Solid Edge part; units mm, degrees
sketch "Sketch1" plane through (0, 0, 0) normal (0, 0, 1) x (1, 0, 0)
  line L0 (-8.89, 16.51) -> (8.89, 16.51)
  line L1 (8.89, 16.51) -> (8.89, -16.51)
  line L2 (8.89, -16.51) -> (-8.89, -16.51)
  line L3 (-8.89, -16.51) -> (-8.89, 16.51)
extrude "Protrusion1" add sketch "Sketch1" along normal blind 1.5875
sketch "Sketch2" plane through (0, 0, 1.5875) normal (0, 0, 1) x (1, 0, 0)
  circle A0 centre (7.62, -15.24) radius 0.4445
  circle A1 centre (4.572, -8.89) radius 0.4445
  circle A2 centre (4.572, -5.9055) radius 0.4445
  circle A3 centre (4.572, 1.27) radius 0.4445
  circle A4 centre (4.572, 3.81) radius 0.4445
  circle A5 centre (7.62, 12.5407) radius 0.4445
  circle A6 centre (6.35, 15.24) radius 0.4445
  circle A7 centre (-6.35, 15.24) radius 0.4445
  circle A8 centre (-7.62, 12.7) radius 0.4445
  circle A9 centre (-7.62, -15.24) radius 0.4445
extrude "Cutout1" cut sketch "Sketch2" against normal through all
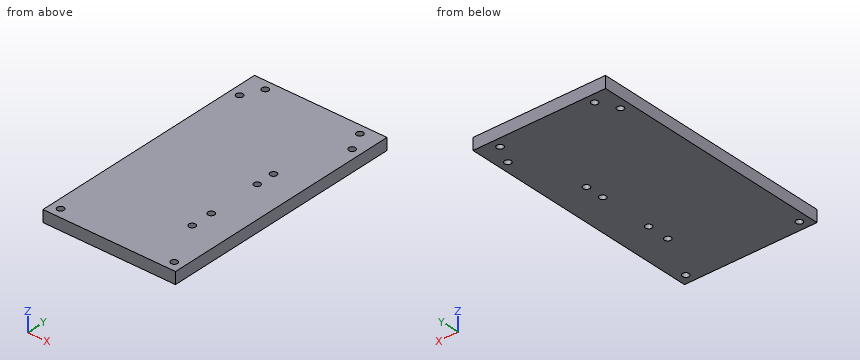
Build history of the part. All positions in model axes, mm. Round coordinates to 2 decimals unless told otherwise and drop trailing zeros. Loops run counter-clockwise (first coordinate to the right, second up) from the corner with the lowest first, then second, coordinate; pieces in that order, holes last. Notation, with made-up numbers: (87.25, -14.5) -> (111.25, -14.5) arc R23 ccw to (111.25, 8.5) -> close; hole circle Ø3 at (74, 20.5). An arc over 180 degrees is marked (long way). One line per item, written item: value. Start each with the question number.
Q1. Cut at B-B on y = 15.24. List the corners of the cut face in (x, z), plus the area to 3 significant figures.
Q2. Cut at A-A on x = 7.62. List the corners of the cut face in (y, z).
Q3. Probe line 1 along Y through (x, z) = (7.62, 0.55); line 2 along Y through (x, z) = (-7.62, 1.2); line 3 along Y through (x, z) = (-6.35, 0.8). List the from-to ranges inside material, lowest first.
Q4. Cut at C-C on y = -8.89. List the corners of the cut face in (x, z).
Computed:
1. outline: (-8.89, 0) -> (-6.79, 0) -> (-6.79, 1.59) -> (-8.89, 1.59) -> close; (-5.91, 0) -> (5.91, 0) -> (5.91, 1.59) -> (-5.91, 1.59) -> close; (6.79, 0) -> (8.89, 0) -> (8.89, 1.59) -> (6.79, 1.59) -> close
1. area: 25.4 mm²
2. outline: (-16.51, 0) -> (-15.68, 0) -> (-15.68, 1.59) -> (-16.51, 1.59) -> close; (-14.8, 0) -> (12.1, 0) -> (12.1, 1.59) -> (-14.8, 1.59) -> close; (12.99, 0) -> (16.51, 0) -> (16.51, 1.59) -> (12.99, 1.59) -> close
3. line 1: -16.51 to -15.68, -14.8 to 12.1, 12.99 to 16.51
3. line 2: -16.51 to -15.68, -14.8 to 12.26, 13.14 to 16.51
3. line 3: -16.51 to 14.8, 15.68 to 16.51
4. outline: (-8.89, 0) -> (4.13, 0) -> (4.13, 1.59) -> (-8.89, 1.59) -> close; (5.02, 0) -> (8.89, 0) -> (8.89, 1.59) -> (5.02, 1.59) -> close
